from build123d import *

# Parameters (mm, degrees)
BOSS_EXTRU_2_DEPTH       = 60
ESQUISSE2_W              = 5
ESQUISSE2_H              = 30
ESQUISSE2_H_2            = 20
ESQUISSE2_W_2            = 25
ENL_V_MAT_EXTRU_1_DEPTH  = 20
ESQUISSE4_W              = 60
ESQUISSE4_H              = 5
ENL_V_MAT_EXTRU_2_DEPTH  = 45
ESQUISSE5_W              = 56.25
ESQUISSE5_H              = 5
ESQUISSE5_W_2            = 3.75
ENL_V_MAT_EXTRU_4_DEPTH  = 27.5
ESQUISSE6_W              = 60
ESQUISSE6_H              = 2.5
BOSS_EXTRU_3_DEPTH       = 29.5
ESQUISSE7_W              = 3.75
ESQUISSE7_H              = 20
ESQUISSE7_W_2            = 13.75
BOSS_EXTRU_4_DEPTH       = 27.5
ESQUISSE8_W              = 3.75
ESQUISSE8_H              = 20
ESQUISSE8_W_2            = 13.75
BOSS_EXTRU_5_DEPTH       = 31.5
ESQUISSE10_W             = 42.5
ESQUISSE10_H             = 5
ENL_V_MAT_EXTRU_5_DEPTH  = 47.5
ESQUISSE11_W             = 5
ESQUISSE11_H             = 2.5
ESQUISSE11_W_2           = 3.75
ESQUISSE11_W_3           = 25
BOSS_EXTRU_6_DEPTH       = 20.5
ESQUISSE13_W             = 42.5
ESQUISSE13_H             = 5
ENL_V_MAT_EXTRU_7_DEPTH  = 27.5
ESQUISSE14_W             = 5
ESQUISSE14_H             = 10
ENL_V_MAT_EXTRU_8_DEPTH  = 40
ESQUISSE15_W             = 5
ESQUISSE15_H             = 20
BOSS_EXTRU_7_DEPTH       = 41
ESQUISSE16_W             = 5
ESQUISSE16_H             = 10
ENL_V_MAT_EXTRU_9_DEPTH  = 30
ESQUISSE17_W             = 5
ESQUISSE17_H             = 43.25
ENL_V_MAT_EXTRU_10_DEPTH = 23.25
ESQUISSE18_W             = 43.75
ESQUISSE18_H             = 0.75
BOSS_EXTRU_8_DEPTH       = 50
ESQUISSE19_W             = 48.75
ESQUISSE19_H             = 4.25
BOSS_EXTRU_9_DEPTH       = 50
ESQUISSE20_W             = 53.75
ESQUISSE20_H             = 5
ENL_V_MAT_EXTRU_11_DEPTH = 23
ESQUISSE21_W             = 53.677626311
ESQUISSE21_H             = 5
ENL_V_MAT_EXTRU_12_DEPTH = 48
ESQUISSE22_W             = 53.677626311
ESQUISSE22_H             = 5
BOSS_EXTRU_10_DEPTH      = 24


with BuildPart() as part:
    # Esquisse1 → Boss.-Extru.2 (new body)
    with BuildSketch(Plane(origin=(0, 0, 0), x_dir=(0, 0, -1), z_dir=(1, 0, 0))):
        Polygon((-38.339385634, 11.238718482), (-18.339385634, 11.238718482), (-18.339385634, -38.761281518), (-48.339385634, -38.761281518), (-48.339385634, -18.761281518), (-38.339385634, -18.761281518), align=None)
    extrude(amount=BOSS_EXTRU_2_DEPTH)

    # Esquisse2 → Enlèv. mat.-Extru.1 (cut)
    with BuildSketch(Plane.XY.offset(48.339385634)):
        with Locations((6.25, -3.761281518)):
            Rectangle(ESQUISSE2_W, ESQUISSE2_H)
        with Locations((6.25, -28.761281518)):
            Rectangle(ESQUISSE2_W, ESQUISSE2_H_2)
        with Locations((25, -3.761281518)):
            Rectangle(ESQUISSE2_W_2, ESQUISSE2_H)
        with Locations((25, -28.761281518)):
            Rectangle(ESQUISSE2_W_2, ESQUISSE2_H_2)
        with Locations((43.75, -3.761281518)):
            Rectangle(ESQUISSE2_W, ESQUISSE2_H)
        with Locations((43.75, -28.761281518)):
            Rectangle(ESQUISSE2_W, ESQUISSE2_H_2)
    extrude(amount=-ENL_V_MAT_EXTRU_1_DEPTH, mode=Mode.SUBTRACT)

    # Esquisse4 → Enlèv. mat.-Extru.2 (cut)
    with BuildSketch(Plane(origin=(0, 11.238718482, 0), x_dir=(1, 0, 0), z_dir=(0, 1, 0))):
        with Locations((30, -23.339385634)):
            Rectangle(ESQUISSE4_W, ESQUISSE4_H)
    extrude(amount=-ENL_V_MAT_EXTRU_2_DEPTH, mode=Mode.SUBTRACT)

    # Esquisse5 → Enlèv. mat.-Extru.4 (cut)
    with BuildSketch(Plane.XY.offset(48.339385634)):
        with Locations((31.875, -33.761281518)):
            Rectangle(ESQUISSE5_W, ESQUISSE5_H)
        with Locations((1.875, -33.761281518)):
            Rectangle(ESQUISSE5_W_2, ESQUISSE5_H)
    extrude(amount=-ENL_V_MAT_EXTRU_4_DEPTH, mode=Mode.SUBTRACT)

    # Esquisse6 → Boss.-Extru.3 (add)
    with BuildSketch(Plane.XY.offset(48.339385634)):
        with Locations((30, -37.511281518)):
            Rectangle(ESQUISSE6_W, ESQUISSE6_H)
    extrude(amount=-BOSS_EXTRU_3_DEPTH)

    # Esquisse7 → Boss.-Extru.4 (add)
    with BuildSketch(Plane.XY.offset(48.339385634)):
        with Locations((1.875, -28.761281518)):
            Rectangle(ESQUISSE7_W, ESQUISSE7_H)
        with Locations((10.625, -28.761281518)):
            Rectangle(ESQUISSE7_W, ESQUISSE7_H)
        with Locations((53.125, -28.761281518)):
            Rectangle(ESQUISSE7_W_2, ESQUISSE7_H)
        with Locations((39.375, -28.761281518)):
            Rectangle(ESQUISSE7_W, ESQUISSE7_H)
    extrude(amount=-BOSS_EXTRU_4_DEPTH)

    # Esquisse8 → Boss.-Extru.5 (add)
    with BuildSketch(Plane(origin=(0, 11.238718482, 0), x_dir=(1, 0, 0), z_dir=(0, 1, 0))):
        with Locations((1.875, -28.339385634)):
            Rectangle(ESQUISSE8_W, ESQUISSE8_H)
        with Locations((10.625, -28.339385634)):
            Rectangle(ESQUISSE8_W, ESQUISSE8_H)
        with Locations((53.125, -28.339385634)):
            Rectangle(ESQUISSE8_W_2, ESQUISSE8_H)
        with Locations((39.375, -28.339385634)):
            Rectangle(ESQUISSE8_W, ESQUISSE8_H)
    extrude(amount=-BOSS_EXTRU_5_DEPTH)

    # Esquisse10 → Enlèv. mat.-Extru.5 (cut)
    with BuildSketch(Plane(origin=(0, 11.238718482, 0), x_dir=(1, 0, 0), z_dir=(0, 1, 0))):
        with Locations((25, -23.339385634)):
            Rectangle(ESQUISSE10_W, ESQUISSE10_H)
    extrude(amount=-ENL_V_MAT_EXTRU_5_DEPTH, mode=Mode.SUBTRACT)

    # Esquisse11 → Boss.-Extru.6 (add)
    with BuildSketch(Plane.XY.offset(48.339385634)):
        with Locations((43.75, -30.011281518)):
            Rectangle(ESQUISSE11_W, ESQUISSE11_H)
        with Locations((39.375, -30.011281518)):
            Rectangle(ESQUISSE11_W_2, ESQUISSE11_H)
        with Locations((25, -30.011281518)):
            Rectangle(ESQUISSE11_W_3, ESQUISSE11_H)
        with Locations((6.25, -30.011281518)):
            Rectangle(ESQUISSE11_W, ESQUISSE11_H)
        with Locations((10.625, -30.011281518)):
            Rectangle(ESQUISSE11_W_2, ESQUISSE11_H)
    extrude(amount=-BOSS_EXTRU_6_DEPTH)

    # Esquisse13 → Enlèv. mat.-Extru.7 (cut)
    with BuildSketch(Plane.XY.offset(48.339385634)):
        with Locations((25, -33.761281518)):
            Rectangle(ESQUISSE13_W, ESQUISSE13_H)
    extrude(amount=-ENL_V_MAT_EXTRU_7_DEPTH, mode=Mode.SUBTRACT)

    # Esquisse14 → Enlèv. mat.-Extru.8 (cut)
    with BuildSketch(Plane(origin=(0, 11.238718482, 0), x_dir=(1, 0, 0), z_dir=(0, 1, 0))):
        with Locations((55, -33.339385634)):
            Rectangle(ESQUISSE14_W, ESQUISSE14_H)
        with Locations((55, -43.339385634)):
            Rectangle(ESQUISSE14_W, ESQUISSE14_H)
    extrude(amount=-ENL_V_MAT_EXTRU_8_DEPTH, mode=Mode.SUBTRACT)

    # Esquisse15 → Boss.-Extru.7 (add)
    with BuildSketch(Plane(origin=(0, 11.238718482, 0), x_dir=(1, 0, 0), z_dir=(0, 1, 0))):
        with Locations((43.75, -38.339385634)):
            Rectangle(ESQUISSE15_W, ESQUISSE15_H)
    extrude(amount=-BOSS_EXTRU_7_DEPTH)

    # Esquisse16 → Enlèv. mat.-Extru.9 (cut)
    with BuildSketch(Plane(origin=(0, 11.238718482, 0), x_dir=(1, 0, 0), z_dir=(0, 1, 0))):
        with Locations((43.75, -43.339385634)):
            Rectangle(ESQUISSE16_W, ESQUISSE16_H)
    extrude(amount=-ENL_V_MAT_EXTRU_9_DEPTH, mode=Mode.SUBTRACT)

    # Esquisse17 → Enlèv. mat.-Extru.10 (cut)
    with BuildSketch(Plane.XY.offset(48.339385634)):
        with Locations((55, -10.386281518)):
            Rectangle(ESQUISSE17_W, ESQUISSE17_H)
        with Locations((6.25, -10.386281518)):
            Rectangle(ESQUISSE17_W, ESQUISSE17_H)
    extrude(amount=-ENL_V_MAT_EXTRU_10_DEPTH, mode=Mode.SUBTRACT)

    # Esquisse18 → Boss.-Extru.8 (add)
    with BuildSketch(Plane(origin=(0, 11.238718482, 0), x_dir=(1, 0, 0), z_dir=(0, 1, 0))):
        with Locations((30.625, -25.464385634)):
            Rectangle(ESQUISSE18_W, ESQUISSE18_H)
    extrude(amount=-BOSS_EXTRU_8_DEPTH)

    # Esquisse19 → Boss.-Extru.9 (add)
    with BuildSketch(Plane(origin=(0, 11.238718482, 0), x_dir=(1, 0, 0), z_dir=(0, 1, 0))):
        with Locations((28.125, -22.964385634)):
            Rectangle(ESQUISSE19_W, ESQUISSE19_H)
    extrude(amount=-BOSS_EXTRU_9_DEPTH)

    # Esquisse20 → Enlèv. mat.-Extru.11 (cut)
    with BuildSketch(Plane.XY.offset(48.339385634)):
        with Locations((30.625, -33.761281518)):
            Rectangle(ESQUISSE20_W, ESQUISSE20_H)
    extrude(amount=-ENL_V_MAT_EXTRU_11_DEPTH, mode=Mode.SUBTRACT)

    # Esquisse21 → Enlèv. mat.-Extru.12 (cut)
    with BuildSketch(Plane(origin=(0, 11.238718482, 0), x_dir=(1, 0, 0), z_dir=(0, 1, 0))):
        with Locations((30.661186845, -21.828072333)):
            Rectangle(ESQUISSE21_W, ESQUISSE21_H)
    extrude(amount=-ENL_V_MAT_EXTRU_12_DEPTH, mode=Mode.SUBTRACT)

    # Esquisse22 → Boss.-Extru.10 (add)
    with BuildSketch(Plane(origin=(0, -36.761281518, 0), x_dir=(1, 0, 0), z_dir=(0, 1, 0))):
        with Locations((30.661186845, -21.828072333)):
            Rectangle(ESQUISSE22_W, ESQUISSE22_H)
    extrude(amount=BOSS_EXTRU_10_DEPTH)


solid = part.part
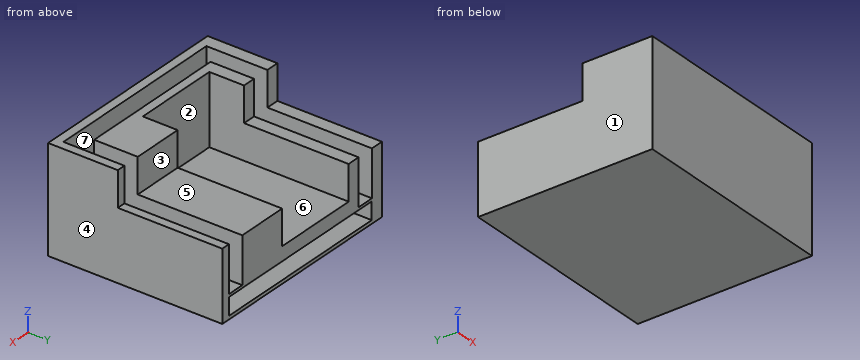
Model file for the job. Use its own axes, mm. Face numbers are marked on the shaded views. A direction names the side the tool comes from. Give positions to 0.01 mm unless a question says otherwise; leave off trailing zeros. Loops run counter-clockwise (first coordinate to the right, second up) from the corner with the lowest first, then second, coordinate; pieces in that order, holes last. Notation, with made-up numbers: (-6.75, 59) - (33.25, 59) arc R26 ccw to (33.25, 92) - close; hole circle Ø11 at (22.5, 80.5). An arc over 180 degrees is marked (long way). Use one line per item in the form item = value.
(1) Drop flat-ended pins along their axis: P1, Ø11.5, axis at y = -17.5, z = 39, coming from the +X side; P2, Ø1.5, axis at x = 23, y = -4.5, coming from the +Z side; P3, Ø2, axis at x = 49.5, y = -4, coming from the +Z side; P4, Ø8, axis at x = 43, z = 45.5, coming from the +Y side. Give the stop position or say it passes through.
Determined:
P1 = 60
P2 = 28.34
P3 = 38.34
P4 = -18.76
(2) Cut at A-A (z = 27.5). Give the cut face in (x, y).
Determined:
outline = (0, -38.76) - (60, -38.76) - (60, 11.24) - (57.5, 11.24) - (57.5, -36.26) - (3.75, -36.26) - (3.75, 11.24) - (0, 11.24) - close; (8.75, -31.26) - (52.5, -31.26) - (52.5, 11.24) - (8.75, 11.24) - close
(3) Cut at C-C (x = 28). Give the cut face in (y, z).
Determined:
outline = (-38.76, 18.34) - (11.24, 18.34) - (11.24, 19.33) - (-12.76, 19.33) - (-12.76, 24.33) - (11.24, 24.33) - (11.24, 28.34) - (-28.76, 28.34) - (-28.76, 48.34) - (-31.26, 48.34) - (-31.26, 25.34) - (-36.26, 25.34) - (-36.26, 48.34) - (-38.76, 48.34) - close
(4) Pull direction X, two halves, no side cores. Call the marked faces 1, 2 and 3: pulls with the +X half, pulls with the -X half, needs draft (parallel to the pull), parting line crosses it, or undercut.
Determined:
face_1 = pulls with the -X half
face_2 = undercut
face_3 = needs draft
(5) Cut at B-B (y = -1.5). Give the cut face in (x, z), then the cut area to 3 significant figures.
Determined:
outline = (0, 18.34) - (60, 18.34) - (60, 38.34) - (57.5, 38.34) - (57.5, 25.09) - (52.5, 25.09) - (52.5, 38.34) - (37.5, 38.34) - (37.5, 28.34) - (12.5, 28.34) - (12.5, 38.34) - (8.75, 38.34) - (8.75, 25.09) - (3.75, 25.09) - (3.75, 38.34) - (0, 38.34) - close; hole (3.82, 19.33) - (57.5, 19.33) - (57.5, 24.33) - (3.82, 24.33) - close
area = 549 mm^2
(6) Cut at D-D (y = -22). Give the cut face in (x, z), then the cut area to 3 significant figures.
Determined:
outline = (0, 18.34) - (60, 18.34) - (60, 48.34) - (57.5, 48.34) - (57.5, 25.09) - (52.5, 25.09) - (52.5, 48.34) - (37.5, 48.34) - (37.5, 28.34) - (12.5, 28.34) - (12.5, 48.34) - (8.75, 48.34) - (8.75, 25.09) - (3.75, 25.09) - (3.75, 48.34) - (0, 48.34) - close
area = 1,070 mm^2
(7) Drill centre lines: L1, parallel to X at y = 6, z = 38; L2, parallel to X at y = -30, z = 29; L3, parallel to Y at x = 48.5, z = 29.5. Where is each one in solid material? Low to high.
Determined:
L1 = 0 to 3.75, 8.75 to 12.5, 37.5 to 52.5, 57.5 to 60
L2 = 0 to 3.75, 8.75 to 52.5, 57.5 to 60
L3 = -38.76 to -36.26, -31.26 to 11.24
(8) 3-axis set-ups, long thin cutter, end or side, ignore diameter. For the marked faces 4, 5, 6 and 7: which of +Z, -Z, +X, -X, +Y, -Y reach the whole face in a straight line?
Determined:
face_4 = +Z, -Z, +X, +Y, -Y
face_5 = +Z, +X, -X, +Y
face_6 = +Z, +Y
face_7 = +Z
